Could you check a few things on this model? Use its own coordinates, in mm. A direction names the side the tool comes from. Coordinates: 2 decimals unless noted, no trailing zeros. Order: outer loops, then holes, each group sorted by start corner. A loop starts at its lowest first (then second) coordinate and runs counter-clockwise, first axis right, second up.
```python
from build123d import *

# Parameters (mm, degrees)
BOSS_EXTRUDE1_DEPTH     = 63.5
SKETCH2_W               = 165.1
SKETCH2_H               = 25.4
CUT_EXTRUDE1_DEPTH      = 38.1
SKETCH3_W               = 107.95
SKETCH3_H               = 146.05
CUT_EXTRUDE2_DEPTH      = 60.325
SKETCH4_W               = 158.75
SKETCH4_H               = 19.05
CUT_EXTRUDE3_DEPTH      = 22.225
CUT_EXTRUDE5_DEPTH      = 20.32
CUT_EXTRUDE5_DEPTH_BACK = 20.32
SKETCH5_R               = 6.35
SKETCH6_W               = 154.94
SKETCH6_H               = 5.08
CUT_EXTRUDE6_DEPTH      = 10.16
SKETCH8_R               = 3.81
CUT_EXTRUDE8_DEPTH      = 12.7
SKETCH9_R               = 6.35
CUT_EXTRUDE9_DEPTH      = 12.7
SKETCH10_R              = 6.35
CUT_EXTRUDE10_DEPTH     = 12.7


with BuildPart() as part:
    # Sketch1 → Boss-Extrude1 (new body)
    with BuildSketch(Plane(origin=(0, 0, 0), x_dir=(1, 0, 0), z_dir=(0, 1, 0))):
        Polygon((-82.55, 12.7), (82.55, 12.7), (196.85, 12.7), (196.85, -139.7), (82.55, -139.7), (82.55, -12.7), (-82.55, -12.7), align=None)
    extrude(amount=BOSS_EXTRUDE1_DEPTH)

    # Sketch2 → Cut-Extrude1 (cut)
    with BuildSketch(Plane(origin=(0, 63.5, 0), x_dir=(1, 0, 0), z_dir=(0, 1, 0))):
        Rectangle(SKETCH2_W, SKETCH2_H)
    extrude(amount=-CUT_EXTRUDE1_DEPTH, mode=Mode.SUBTRACT)

    # Sketch3 → Cut-Extrude2 (cut)
    with BuildSketch(Plane(origin=(0, 63.5, 0), x_dir=(1, 0, 0), z_dir=(0, 1, 0))):
        with Locations((139.7, -63.5)):
            Rectangle(SKETCH3_W, SKETCH3_H)
    extrude(amount=-CUT_EXTRUDE2_DEPTH, mode=Mode.SUBTRACT)

    # Sketch4 → Cut-Extrude3 (cut)
    with BuildSketch(Plane(origin=(0, 25.4, 0), x_dir=(1, 0, 0), z_dir=(0, 1, 0))):
        Rectangle(SKETCH4_W, SKETCH4_H)
    extrude(amount=-CUT_EXTRUDE3_DEPTH, mode=Mode.SUBTRACT)

    # Sketch5 → Cut-Extrude5 (cut, two sides: drawn at the far end of the back side and taken through both)
    with BuildSketch(Plane.ZY.offset(-79.375).offset(-CUT_EXTRUDE5_DEPTH_BACK)):
        with Locations(Location((0, 15.24, 0), (0, 0, 180))):
            Circle(SKETCH5_R)
    extrude(amount=CUT_EXTRUDE5_DEPTH + CUT_EXTRUDE5_DEPTH_BACK, mode=Mode.SUBTRACT)

    # Sketch6 → Cut-Extrude6 (cut)
    with BuildSketch(Plane.XY.offset(12.7)):
        with Locations((0, 12.7)):
            Rectangle(SKETCH6_W, SKETCH6_H)
    extrude(amount=-CUT_EXTRUDE6_DEPTH, mode=Mode.SUBTRACT)

    # Sketch8 → Cut-Extrude8 (cut)
    with BuildSketch(Plane.ZY.offset(-82.55)):
        with Locations((57.15, 16.51)):
            Circle(SKETCH8_R)
        with Locations((77.47, 16.51)):
            Circle(SKETCH8_R)
        with Locations((97.79, 16.51)):
            Circle(SKETCH8_R)
    extrude(amount=-CUT_EXTRUDE8_DEPTH, mode=Mode.SUBTRACT)

    # Sketch9 → Cut-Extrude9 (cut)
    with BuildSketch(Plane.XY.offset(139.7)):
        with Locations((180.34, 16.51)):
            Circle(SKETCH9_R)
    extrude(amount=-CUT_EXTRUDE9_DEPTH, mode=Mode.SUBTRACT)

    # Sketch10 → Cut-Extrude10 (cut)
    with BuildSketch(Plane(origin=(196.85, 0, 0), x_dir=(0, 0, -1), z_dir=(1, 0, 0))):
        with Locations((-123.19, 16.51)):
            Circle(SKETCH10_R)
    extrude(amount=-CUT_EXTRUDE10_DEPTH, mode=Mode.SUBTRACT)


solid = part.part
```
Item 1: Thinking about a two-plate mould opening in Y: for faces 1 (the face through (173.996, 16.789, 138.135)), 2 (the face through (139, 34, -9.525)), 3 (the face through (-13, 25.4, 10)), which applies, +Y half, -Y half, draft (parallel to the pull), parting line (faces both ways), or undercut?
Item 2: Suppose I cut it at A-A (z = 57.15). List the corners of the cut face in (x, y) for me (3 decimals), and give its area (3 significant figures).
Item 3: Suppose I cut it at D-D (z = 123.19). List the corners of the cut face in (x, y) for me (3 decimals).
Item 4: Which directions (+Z, -Z, +X, -X, +Y, -Y) give clear straight access to the entire face, cutting with the end or side of a thin tool? Please do faces 4 (the face through (84.12, 19.08, 54.34)), 5 (the face through (1, 10, 12.7)), 6 (the face through (82.594, 8.944, 0.827)), 7 (the face through (85.725, 34, 65)).
Item 5: I need wall thicknesses on line 1 (Y direction, x = 81.75, z = 0); line 2 (X direction, y = 6.5, z = 98) (3 decimals); line 3 (Z direction, x = -38, y = 8) (3 decimals). Which ranges of each line are inside material? Lowest first, please.
Item 6: Suppose I cut it at B-B (y = 29). List the corners of the cut face in (x, z) for me (3 decimals).
Item 7: For pin 1 Ø1 at (y, z) = (43.5, 120.5) entering from -X; pin 2 Ø2.5 at (x, z) = (-8, 10.5) entering from +Y; pin 3 Ø7.5 at (x, y) = (-29.5, 13) entering from +Z, each with a flat end and sliding along its axis, tell me the tip position at first contact or that it passes through.
Item 8: Suppose I cut it at C-C (x = 131). List the corners of the cut face in (y, z) for me (3 decimals), and give its area (3 significant figures).
Geometry results:
1. face 1: undercut
1. face 2: draft
1. face 3: +Y half
2. outline: (82.55, 0) - (196.85, 0) - (196.85, 63.5) - (193.675, 63.5) - (193.675, 3.175) - (85.725, 3.175) - (85.725, 12.7) - (82.55, 12.7) - close; (82.55, 20.32) - (85.725, 20.32) - (85.725, 63.5) - (82.55, 63.5) - close
2. area: 722 mm2
3. outline: (82.55, 0) - (196.85, 0) - (196.85, 10.16) - (193.675, 10.16) - (193.675, 3.175) - (85.725, 3.175) - (85.725, 63.5) - (82.55, 63.5) - close; (193.675, 22.86) - (196.85, 22.86) - (196.85, 63.5) - (193.675, 63.5) - close
4. face 4: -X
4. face 5: +Z, -X, +Y, -Y
4. face 6: none
4. face 7: +Y
5. line 1: y = 0 to 8.89, 21.59 to 25.4
5. line 2: x = 82.55 to 85.725, 193.675 to 196.85
5. line 3: z = -12.7 to -9.525, 9.525 to 12.7
6. outline: (82.55, -12.7) - (196.85, -12.7) - (196.85, 139.7) - (82.55, 139.7) - close; hole (85.725, -9.525) - (193.675, -9.525) - (193.675, 136.525) - (85.725, 136.525) - close
7. pin 1: stops at x = 82.55
7. pin 2: stops at y = 25.4
7. pin 3: stops at z = 12.7
8. outline: (0, -12.7) - (63.5, -12.7) - (63.5, -9.525) - (3.175, -9.525) - (3.175, 136.525) - (63.5, 136.525) - (63.5, 139.7) - (0, 139.7) - close
8. area: 867 mm2
